For this review, take the finished solid that the model builds, in its own axes (mm). Face numbers are marked on the shaded views. A direction names the side the tool comes from. Give positions to 0.01 mm unless a question says otherwise; leave off trailing zeros. Loops run counter-clockwise (first coordinate to the right, second up) from the corner with the lowest first, then second, coordinate; pieces in that order, holes last.
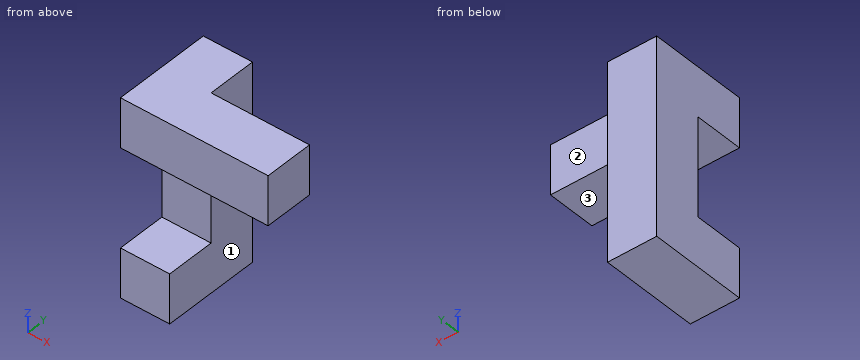
```python
from build123d import *

# Parameters (mm, degrees)
F1_DEPTH = 25.4
F2_W     = 25.4
F2_H     = 25.4
F3_DEPTH = 50.8


with BuildPart() as f1:
    # F0 (on Right) → F1 (new body)
    with BuildSketch(Plane.YZ):
        Polygon((50.8, 101.6), (0, 101.6), (0, 76.2), (25.4, 76.2), (25.4, 25.4), (0, 25.4), (0, 0), (50.8, 0), align=None)
    extrude(amount=F1_DEPTH)

    # F2 (on face) → F3 (join)
    with BuildSketch(Plane.YZ.offset(25.4)):
        with Locations((12.7, 88.9)):
            Rectangle(F2_W, F2_H)
    extrude(amount=F3_DEPTH)


solid = f1.part
```
Item 1: Take a section at D-D on y = 39.5. Give the boundary of the cut face in (x, z), and give its area (3 significant figures).
Answer:
outline: (0, 0) - (25.4, 0) - (25.4, 101.6) - (0, 101.6) - close
area: 2,580 mm2
Item 2: Take a section at C-C on x = 14. Give the boundary of the cut face in (y, z), and give its area (3 significant figures).
Answer:
outline: (0, 0) - (50.8, 0) - (50.8, 101.6) - (0, 101.6) - (0, 76.2) - (25.4, 76.2) - (25.4, 25.4) - (0, 25.4) - close
area: 3,870 mm2
Item 3: Tool access review of the marked faces 1, 2 and 3: name each direction out of +Z, -Z, +X, -X, +Y, -Y from which nothing blocks a thin tool from reaching the whole face with its end or side.
Answer:
face 1: -Z, +X, +Y
face 2: +Z, -Z, +X, +Y
face 3: +X, -X, -Y
Item 4: Clearance check with flat-ended pins moving along their axes: pin 1 Ø1.5 at (y, z) = (26.5, 87) entering from +X; pin 2 Ø12.5 at (x, z) = (14.5, 52.5) entering from -Y. State where each tip first meets the part, or that it passes through.
Answer:
pin 1: stops at x = 25.4
pin 2: stops at y = 25.4
Item 5: For L1, parallel to Z at x = 14, y = 6; L2, parallel to X at y = 35, z = 13; L3, parallel to Z at x = 49, y = 18, list the stretches that pass through material, from the lowest coordinate up.
Answer:
L1: z = 0 to 25.4, 76.2 to 101.6
L2: x = 0 to 25.4
L3: z = 76.2 to 101.6
Item 6: Take a section at A-A on y = 18.5. Give the boundary of the cut face in (x, z).
Answer:
outline: (0, 0) - (25.4, 0) - (25.4, 25.4) - (0, 25.4) - close; (0, 76.2) - (76.2, 76.2) - (76.2, 101.6) - (0, 101.6) - close
Item 7: Take a section at B-B on z = 83.5. Give the boundary of the cut face in (x, y), and give its area (3 significant figures).
Answer:
outline: (0, 0) - (76.2, 0) - (76.2, 25.4) - (25.4, 25.4) - (25.4, 50.8) - (0, 50.8) - close
area: 2,580 mm2
